The listing builds one solid part. Answer for the finished solid, in the listing's coordinates (mm). A direction names the side the tool comes from. Round coordinates to 2 decimals unless told otherwise and drop trailing zeros. Order: outer loops, then holes, each group sorted by start corner. A loop starts at its lowest first (then second) coordinate and runs counter-clockwise, first axis right, second up. Notation, with made-up numbers: (70, 15) -> (78, 15) arc R22 cw to (78, 29) -> close; hole circle Ø1 at (-32, 68). An arc over 180 degrees is marked (long way). Answer in a Markdown table with one row per item. Add a question column.
```python
from build123d import *

# Parameters (mm, degrees)
SKETCH034_R     = 3.0625
PAD004_DEPTH    = 27.5
SKETCH_R        = 1.6
POCKET_DEPTH    = 5
POCKET021_DEPTH = 2
SKETCH036_W     = 26
SKETCH036_H     = 8
POCKET022_DEPTH = 14
SKETCH037_W     = 10
SKETCH037_H     = 5.5
PAD005_DEPTH    = 5
SKETCH038_R     = 1.6
POCKET023_DEPTH = 8.5
SKETCH039_W     = 6.5
SKETCH039_H     = 2.5
POCKET024_DEPTH = 6.5
SKETCH040_W     = 6.5
SKETCH040_H     = 2.5
POCKET025_DEPTH = 6.5
SKETCH041_W     = 17
SKETCH041_H     = 14
POCKET026_DEPTH = 9
FILLET_R        = 1
FILLET001_R     = 3


with BuildPart() as part:
    # Sketch034 → Pad004 (new body)
    with BuildSketch(Plane.XZ):
        Polygon((33, -7), (33, 2), (75, 2), (75, 7), (-75, 7), (-75, 2), (-33, 2), (-33, -7), (-7, -7), (-7, 2), (7, 2), (7, -7), align=None)
        with Locations((-14, 0)):
            Circle(SKETCH034_R, mode=Mode.SUBTRACT)
        with Locations((14, 0)):
            Circle(SKETCH034_R, mode=Mode.SUBTRACT)
        with Locations((-26, 0)):
            Circle(SKETCH034_R, mode=Mode.SUBTRACT)
        with Locations((26, 0)):
            Circle(SKETCH034_R, mode=Mode.SUBTRACT)
    extrude(amount=PAD004_DEPTH)

    # Sketch (on Face4 of Pad004) → Pocket (cut)
    with BuildSketch(Plane(origin=(0, 0, 7), x_dir=(-1, 0, 0), z_dir=(0, 0, 1))):
        with Locations((-66.75, 13.75)):
            Circle(SKETCH_R)
        with Locations((66.75, 13.75)):
            Circle(SKETCH_R)
    extrude(amount=-POCKET_DEPTH, mode=Mode.SUBTRACT)

    # Sketch035 (on Face3 of Pocket) → Pocket021 (cut)
    with BuildSketch(Plane(origin=(0, 0, 2), x_dir=(1, 0, 0), z_dir=(0, 0, -1))):
        Polygon((-63.5, 13.75), (-65.125, 16.5645825623), (-68.375, 16.5645825623), (-70, 13.75), (-68.375, 10.9354174377), (-65.125, 10.9354174377), align=None)
        Polygon((70, 13.75), (68.375, 16.5645825623), (65.125, 16.5645825623), (63.5, 13.75), (65.125, 10.9354174377), (68.375, 10.9354174377), align=None)
    extrude(amount=-POCKET021_DEPTH, mode=Mode.SUBTRACT)

    # Sketch036 (on Face14 of Pocket021) → Pocket022 (cut)
    with BuildSketch(Plane(origin=(0, 0, 7), x_dir=(-1, 0, 0), z_dir=(0, 0, 1))):
        with Locations((-20, 13.5)):
            Rectangle(SKETCH036_W, SKETCH036_H)
        with Locations((20, 13.5)):
            Rectangle(SKETCH036_W, SKETCH036_H)
    extrude(amount=-POCKET022_DEPTH, mode=Mode.SUBTRACT)

    # Sketch037 (on Face7 of Pocket022) → Pad005 (join)
    with BuildSketch(Plane(origin=(0, 0, 7), x_dir=(-1, 0, 0), z_dir=(0, 0, 1))):
        with Locations((-27, 24.75)):
            Rectangle(SKETCH037_W, SKETCH037_H)
        with Locations((27, 24.75)):
            Rectangle(SKETCH037_W, SKETCH037_H)
        with Locations((-27, 2.75)):
            Rectangle(SKETCH037_W, SKETCH037_H)
        with Locations((27, 2.75)):
            Rectangle(SKETCH037_W, SKETCH037_H)
    extrude(amount=PAD005_DEPTH)

    # Sketch038 (on Face70 of Pad005) → Pocket023 (cut)
    with BuildSketch(Plane(origin=(0, 0, 12), x_dir=(-1, 0, 0), z_dir=(0, 0, 1))):
        with Locations((-27, 24.625)):
            Circle(SKETCH038_R)
        with Locations((-27, 2.625)):
            Circle(SKETCH038_R)
        with Locations((27, 24.625)):
            Circle(SKETCH038_R)
        with Locations((27, 2.625)):
            Circle(SKETCH038_R)
    extrude(amount=-POCKET023_DEPTH, mode=Mode.SUBTRACT)

    # Sketch039 (on Face2 of Pocket023) → Pocket024 (cut)
    with BuildSketch(Plane(origin=(0, 0, 0), x_dir=(1, 0, 0), z_dir=(0, 1, 0))):
        with Locations((-27, -5.25)):
            Rectangle(SKETCH039_W, SKETCH039_H)
        with Locations((27, -5.25)):
            Rectangle(SKETCH039_W, SKETCH039_H)
    extrude(amount=-POCKET024_DEPTH, mode=Mode.SUBTRACT)

    # Sketch040 (on Face31 of Pocket024) → Pocket025 (cut)
    with BuildSketch(Plane.XZ.offset(27.5)):
        with Locations((-27, 5.25)):
            Rectangle(SKETCH040_W, SKETCH040_H)
        with Locations((27, 5.25)):
            Rectangle(SKETCH040_W, SKETCH040_H)
    extrude(amount=-POCKET025_DEPTH, mode=Mode.SUBTRACT)

    # Sketch041 (on Face2 of Pocket025) → Pocket026 (cut)
    with BuildSketch(Plane(origin=(0, 0, 0), x_dir=(1, 0, 0), z_dir=(0, 1, 0))):
        Rectangle(SKETCH041_W, SKETCH041_H)
    extrude(amount=-POCKET026_DEPTH, mode=Mode.SUBTRACT)

    # Fillet
    fillet_edges = [part.edges().sort_by_distance(p)[0] for p in [
        (8.5, -9, 0),
        (-8.5, -9, 0),
    ]]
    fillet(fillet_edges, radius=FILLET_R)

    # Fillet001
    fillet001_edges = [part.edges().sort_by_distance(p)[0] for p in [
        (7, -9.5, 4.5),
        (-7, -9.5, 4.5),
    ]]
    fillet(fillet001_edges, radius=FILLET001_R)


solid = part.part
```
Item 1: The part is cut by section B-B, the plane x = -15.5. Give the vertices of the cut face in (y, z).
Item 2: The part is cut by section A-A, the plane x = -66.75. Give the vertices of the cut face in (y, z).
Item 3: Find the intervals of material crossed by probe 1 along Y at (x, z) = (27, 3.8) (3 decimals); probe 2 along X at (y, z) = (-6, 0); probe 3 along X at (y, z) = (-23.5, 0), in increasing order. Write a range as [from, to].
Item 4: The part is cut by section D-D, the plane x = 14. Give the vertices of the cut face in (y, z).
Item 5: For a pull along Y with two mould halves and no side action, classify faces 5 (the face through (34, 0, 3)), 6 (the face through (-65, -13, 4)), 7 (the face through (-20, -5, -7)) as released by +Y, released by -Y, zero draft, split by the parting line, or undercut.
Item 6: The part is cut by section C-C, the plane z = 0. State how many separate pieces and enclosed holes the cut face has, and give its area (3 significant figures).
Item 7: A tool of negligible diameter and unlimited length cuts with its end or side. For faces 1 (the face through (65, -13, 4)), 2 (the face through (-27.05, -22.85, 4)), 3 (the face through (8.5, -4, 0)), 4 (the face through (7, -22, -2)), from which of +Z, -Z, +X, -X, +Y, -Y can it reach the whole face along a straight path? Write none if from no direction.
Item 8: Flat-ended cylindrical pins translate along their axes: P1, Ø1.6, axis at x = -27, y = -25, coming from the +Z side; P2, Ø2.5, axis at y = -5, z = -0.5, coming from the -X side; P3, Ø12, axis at x = 56, y = -19.5, coming from the -Z side. Find the tip coordinate at first contact, or state that the pin passes through.
Resolved:
| question | item | result |
|---|---|---|
| 1 | outline | (-27.5, -7) -> (-17.5, -7) -> (-17.5, -2.67) -> (-27.5, -2.67) -> close; (-27.5, 2.67) -> (-17.5, 2.67) -> (-17.5, 7) -> (-27.5, 7) -> close; (-9.5, -7) -> (0, -7) -> (0, -2.67) -> (-9.5, -2.67) -> close; (-9.5, 2.67) -> (0, 2.67) -> (0, 7) -> (-9.5, 7) -> close |
| 2 | outline | (-27.5, 2) -> (-16.56, 2) -> (-16.56, 4) -> (-15.35, 4) -> (-15.35, 7) -> (-27.5, 7) -> close; (-12.15, 4) -> (-10.94, 4) -> (-10.94, 2) -> (0, 2) -> (0, 7) -> (-12.15, 7) -> close |
| 3 | probe 1 | [-27.5, -26.225], [-23.025, -17.5], [-9.5, -4.225], [-1.025, 0] |
| 3 | probe 2 | [-33, -29.06], [-22.94, -17.06], [-10.94, -8.5], [8.5, 10.94], [17.06, 22.94], [29.06, 33] |
| 3 | probe 3 | [-33, -29.06], [-22.94, -17.06], [-10.94, -7], [7, 10.94], [17.06, 22.94], [29.06, 33] |
| 4 | outline | (-27.5, -7) -> (-17.5, -7) -> (-17.5, -3.06) -> (-27.5, -3.06) -> close; (-27.5, 3.06) -> (-17.5, 3.06) -> (-17.5, 7) -> (-27.5, 7) -> close; (-9.5, -7) -> (0, -7) -> (0, -3.06) -> (-9.5, -3.06) -> close; (-9.5, 3.06) -> (0, 3.06) -> (0, 7) -> (-9.5, 7) -> close |
| 5 | face 5 | released by +Y |
| 5 | face 6 | undercut |
| 5 | face 7 | zero draft |
| 6 | separate pieces | 12 |
| 6 | enclosed holes | 0 |
| 6 | area | 510 mm2 |
| 7 | face 1 | -Z |
| 7 | face 2 | -Y |
| 7 | face 3 | +Z, -Z, +Y |
| 7 | face 4 | -Z, +Y, -Y |
| 8 | P1 | z = 3.5 |
| 8 | P2 | x = -33 |
| 8 | P3 | z = 2 |
